Input: part model. Units: mm. Frame: model coordinates. Face numbers are marked on the shaded views. A direction names the side the tool comes from. Round coordinates to 2 decimals unless told otherwise and drop trailing zeros. Loops run counter-clockwise (first coordinate to the right, second up) from the corner with the lowest first, then second, coordinate; pieces in that order, holes last. Notation, with made-up numbers: (50.5, -38) -> (77.5, -38) arc R12 ccw to (77.5, -27) -> close; hole circle Ø3 at (31, 57.5). An arc over 180 degrees is marked (long way). Answer as a JSON object with one key per item and string values.
```python
from build123d import *

# Parameters (mm, degrees)
SKETCH1_W           = 2
SKETCH1_H           = 10
BOSS_EXTRUDE1_DEPTH = 10
BOSS_EXTRUDE2_DEPTH = 5
SKETCH3_R           = 1
CUT_EXTRUDE1_DEPTH  = 15


with BuildPart() as part:
    # Sketch1 → Boss-Extrude1 (new body)
    with BuildSketch(Plane(origin=(0, 0, 0), x_dir=(1, 0, 0), z_dir=(0, 1, 0))):
        with Locations((0.229885057, -3.379310345)):
            Rectangle(SKETCH1_W, SKETCH1_H)
    extrude(amount=BOSS_EXTRUDE1_DEPTH)

    # Sketch2 → Boss-Extrude2 (add)
    with BuildSketch(Plane(origin=(1.229885057, 0, 0), x_dir=(0, 0, -1), z_dir=(1, 0, 0))):
        Polygon((-2.379310345, 4), (-4.379310345, 6), (-5.379310345, 6), (-5.379310345, 4), align=None)
        Polygon((-1.379310345, 6), (-4.379310345, 6), (-2.379310345, 4), (-1.379310345, 4), align=None)
    extrude(amount=BOSS_EXTRUDE2_DEPTH)

    # Sketch3 → Cut-Extrude1 (cut)
    with BuildSketch(Plane(origin=(0, 6, 0), x_dir=(1, 0, 0), z_dir=(0, 1, 0))):
        with Locations((3.229885057, -3.379310345)):
            Circle(SKETCH3_R)
        with BuildLine():
            Line((3.229885057, -1.379310345), (6.229885057, -1.379310345))
            Line((6.229885057, -1.379310345), (6.229885057, -5.379310345))
            Line((6.229885057, -5.379310345), (3.229885057, -5.379310345))
            ThreePointArc((3.229885057, -5.379310345), (5.229885057, -3.379310345), (3.229885057, -1.379310345))
        make_face()
    extrude(amount=-CUT_EXTRUDE1_DEPTH, mode=Mode.SUBTRACT)


solid = part.part
```
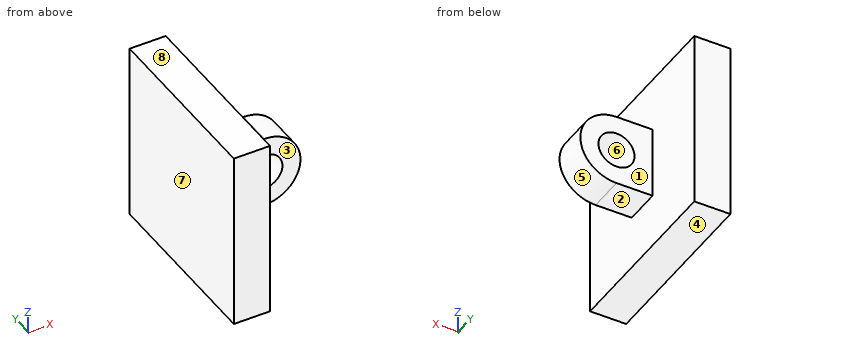
1) Section D-D, the plane x = 1.8. Output: boundary loops of the cut face in (y, z), plus the area to 3 significant figures.
Output:
{"outline": "(4, 1.38) -> (6, 1.38) -> (6, 5.38) -> (4, 5.38) -> close", "area": "8.00 mm^2"}
2) Section B-B, the plane x = 3.05. Output: boundary loops of the cut face in (y, z).
Output:
{"outline": "(4, 1.38) -> (6, 1.38) -> (6, 2.4) -> (4, 2.4) -> close; (4, 4.36) -> (6, 4.36) -> (6, 5.38) -> (4, 5.38) -> close"}
3) Contact query for flat-ended pins moving along their axis: P1, Ø2, axis at x = 3.5, y = 5.5, coming from the -Z side; P2, Ø1.6, axis at x = 2.5, y = 5, coming from the +Z side; P3, Ø2, axis at x = 2.5, z = 3.5, coming from the +Y side. Output: stop coordinate, or through.
Output:
{"P1": "stops at z = 1.38", "P2": "stops at z = 5.38", "P3": "stops at y = 6"}
4) Section C-C, the plane z = 3. Output: boundary loops of the cut face in (x, y).
Output:
{"outline": "(-0.77, 0) -> (1.23, 0) -> (1.23, 4) -> (2.3, 4) -> (2.3, 6) -> (1.23, 6) -> (1.23, 10) -> (-0.77, 10) -> close; (4.16, 4) -> (5.19, 4) -> (5.19, 6) -> (4.16, 6) -> close"}
5) Draft query along Z for the marked faces 6, 7 and 8. Return one class per face: +Z half, -Z half, draft (parallel to the pull), parting line (faces both ways), or undercut.
Output:
{"face 6": "undercut", "face 7": "draft", "face 8": "+Z half"}
6) Ray query, probe 1 along Y at (x, z) = (3.75, 2); probe 2 along Z at (x, y) = (2, 5); probe 3 along X at (y, z) = (2, 1.75). Return the intervals inside material, ascending.
Output:
{"probe 1": "y = 4 to 6", "probe 2": "z = 1.38 to 5.38", "probe 3": "x = -0.77 to 1.23"}
7) Reachability of the marked faces 1, 2, 3, 4 and 5 from +Z, -Z, +X, -X, +Y, -Y: full face, straight path, thin tool, end or side. Return the list, or none.
Output:
{"face 1": "+Z, -Z, +X, +Y", "face 2": "-Z, +X, +Y, -Y", "face 3": "+Z, -Z, +X, -Y", "face 4": "-Z, +X, -X, +Y, -Y", "face 5": "+X, +Y, -Y"}
8) Section A-A, the plane y = 5. Output: boundary loops of the cut face in (x, z).
Output:
{"outline": "(-0.77, -1.62) -> (1.23, -1.62) -> (1.23, 1.38) -> (3.23, 1.38) arc R2 ccw to (3.23, 5.38) -> (1.23, 5.38) -> (1.23, 8.38) -> (-0.77, 8.38) -> close; hole circle Ø2 at (3.23, 3.38)"}
